from build123d import *

# Parameters (mm, degrees)
BOSS_EXTRUDE2_DEPTH = 3


with BuildPart() as part:
    # Sketch1 → Boss-Extrude2 (new body)
    with BuildSketch(Plane.XY):
        Polygon((-28.809910954, -18.295958876), (-31.809910954, -18.295958876), (-16.234936413, -30.842678291), (-16.234936413, -27.842678291), (-6.234936413, -27.842678291), (-6.234936413, -30.842678291), (3.765063587, -30.842678291), (3.765063587, -27.842678291), (13.765063587, -27.842678291), (13.765063587, -30.842678291), (23.765063587, -30.842678291), (23.765063587, -27.842678291), (33.765063587, -27.842678291), (33.765063587, -30.842678291), (62.690506023, 3.62932165), (59.736082763, 3.108377117), (57.999600987, 12.956454647), (60.954024246, 13.47739918), (59.217542469, 23.32547671), (56.26311921, 22.804532177), (54.526637433, 32.652609707), (57.481060693, 33.17355424), (55.744578916, 43.02163177), (52.790155657, 42.500687237), (51.05367388, 52.348764767), (54.008097139, 52.8697093), (33.432510355, 67.069893401), (-31.809910954, 41.704041124), (-28.809910954, 41.704041124), (-28.809910954, 26.704041124), (-31.809910954, 26.704041124), (-31.809910954, 16.704041124), (-28.809910954, 16.704041124), (-28.809910954, 6.704041124), (-31.809910954, 6.704041124), (-31.809910954, -3.295958876), (-28.809910954, -3.295958876), align=None)
    extrude(amount=BOSS_EXTRUDE2_DEPTH)


solid = part.part
Geometry check sheet. Reference: the model listing, model coordinates, mm. A direction names the side the tool comes from. Give positions to 0.01 mm unless a question says otherwise; leave off trailing zeros. Loops run counter-clockwise (first coordinate to the right, second up) from the corner with the lowest first, then second, coordinate; pieces in that order, holes last. Notation, with made-up numbers: (42.5, -11.5) -> (99.5, -11.5) arc R22 cw to (99.5, 8.5) -> close; hole circle Ø3 at (-26.5, -33). An arc over 180 degrees is marked (long way). Answer in a Markdown table with one row per item. Add a question column.
1) Gauge pin test, flat ends, axial feed: P1, Ø0.9, axis at x = 31, z = 1.5, coming from the -Y side; P2, Ø0.9, axis at x = -30, z = 2, coming from the -Y side; P3, Ø0.9, axis at y = -30, z = 1, coming from the -X side. Record the tip position at first contact, or that the pin passes through.
2) Material ranges on probe 1 along X at (y, z) = (32.5, 1.6); probe 2 along X at (y, z) = (-4, 2.9); probe 3 along Y at (x, z) = (-12, 2.65), recorded low to high. Write a range as from..to.
3) Draft check along Y on faces 6 (the face through (19, -30.843, 1)), 7 (the face through (-31.81, 2, 1)), 8 (the face through (-30, 16.704, 1)), 9 (the face through (43.864, 59.87, 1.479)). Enter one of: pulls with the +Y half, pulls with the -Y half, needs draft (parallel to the pull), parting line crosses it, or undercut.
4) Set-up check for faces 1 (the face through (-31.81, 22, 1)), 2 (the face through (55.98, 32.91, 1.48)), 3 (the face through (-28.81, 34, 1)), 4 (the face through (3.765, -29, 1)), 5 (the face through (57.76, 23.07, 1.48)): record each of +Z, -Z, +X, -X, +Y, -Y from which the full face is reachable in a straight line by a thin tool's end or side.
5) Cross-section at B-B on x = 25.5. Record the boundary of the cut face in (y, z), and give its area (3 significant figures).
6) Cross-section at A-A on y = 55. Record the boundary of the cut face in (x, z).
Outcome:
| question | item | result |
|---|---|---|
| 1 | P1 | stops at y = -27.84 |
| 1 | P2 | stops at y = -20.12 |
| 1 | P3 | stops at x = -17.84 |
| 2 | probe 1 | x = -28.81..54.55 |
| 2 | probe 2 | x = -28.81..56.29 |
| 2 | probe 3 | y = -27.84..49.41 |
| 3 | face 6 | pulls with the -Y half |
| 3 | face 7 | needs draft |
| 3 | face 8 | undercut |
| 3 | face 9 | pulls with the +Y half |
| 4 | face 1 | +Z, -Z, -X, +Y, -Y |
| 4 | face 2 | +Z, -Z, +X |
| 4 | face 3 | +Z, -Z, -X |
| 4 | face 4 | +Z, -Z, -Y |
| 4 | face 5 | +Z, -Z |
| 5 | outline | (-27.84, 0) -> (63.99, 0) -> (63.99, 3) -> (-27.84, 3) -> close |
| 5 | area | 275 mm^2 |
| 6 | outline | (2.39, 0) -> (50.92, 0) -> (50.92, 3) -> (2.39, 3) -> close |
